Can you work these out from the model? Positions are in its coordinate system, mm. Face numbers are marked on the shaded views. A direction names the side the tool comes from. Give positions to 0.01 mm unless a question says otherwise; leave off trailing zeros. Order: outer loops, then holes, each group sorted by start corner. A loop starts at its lowest first (then second) coordinate and runs counter-clockwise, first axis right, second up. Notation, with made-up numbers: (82, -32) -> (106, -32) arc R19 cw to (106, 3) -> close; hole circle Ø8 at (-20, 23). An arc over 180 degrees is marked (long way). Answer as a JSON object with one key per item and string values.
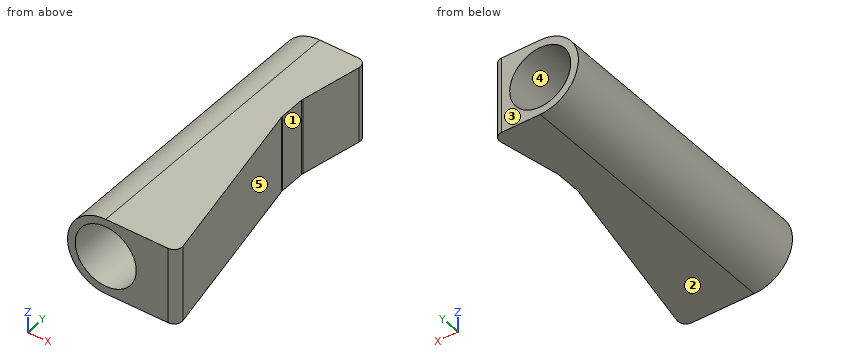
```python
from build123d import *

# Parameters (mm, degrees)
SKETCH1_R           = 14.2875
SKETCH1_R_2         = 11.4125
BOSS_EXTRUDE1_DEPTH = 152.4
SKETCH2_W           = 28.575
SKETCH2_H           = 152.4
BOSS_EXTRUDE2_DEPTH = 12.7
BOSS_EXTRUDE3_DEPTH = 152.4
CUT_EXTRUDE1_DEPTH  = 29.575
FILLET1_R           = 3
SKETCH6_W           = 50
SKETCH6_H           = 45
CUT_EXTRUDE2_DEPTH  = 82
FILLET2_R           = 3


with BuildPart() as part:
    # Sketch1 → Boss-Extrude1 (new body)
    with BuildSketch(Plane(origin=(0, 0, 0), x_dir=(1, 0, 0), z_dir=(0, 1, 0))):
        Circle(SKETCH1_R)
        Circle(SKETCH1_R_2, mode=Mode.SUBTRACT)
    extrude(amount=BOSS_EXTRUDE1_DEPTH)



with BuildPart() as body_2:
    # Sketch2 → Boss-Extrude2 (new body)
    with BuildSketch(Plane(origin=(14.2875, 0, 0), x_dir=(0, 0, -1), z_dir=(1, 0, 0))):
        with Locations((0, 76.2)):
            Rectangle(SKETCH2_W, SKETCH2_H)
    extrude(amount=BOSS_EXTRUDE2_DEPTH)


with BuildPart() as part_1:
    add(part.part)

    add(body_2.part)  # Boss-Extrude3 merges body 2
    # Sketch3 → Boss-Extrude3 (add, through all)
    with BuildSketch(Plane(origin=(0, 152.4, 0), x_dir=(1, 0, 0), z_dir=(0, 1, 0))):
        with BuildLine():
            Line((14.2875, -14.2875), (0, -14.2875))
            ThreePointArc((0, -14.2875), (14.2875, 0), (0, 14.2875))
            Line((0, 14.2875), (14.2875, 14.2875))
            Line((14.2875, 14.2875), (26.9875, 14.2875))
            Line((26.9875, 14.2875), (26.9875, -14.2875))
            Line((26.9875, -14.2875), (14.2875, -14.2875))
        make_face()
    extrude(amount=-BOSS_EXTRUDE3_DEPTH)

    # Sketch5 → Cut-Extrude1 (cut, through all)
    with BuildSketch(Plane.XY.offset(14.2875)):
        Polygon((26.9875, 0), (12.897222949, 71.2), (12.897222949, 81.2), (26.9875, 152.4), align=None)
    extrude(amount=-CUT_EXTRUDE1_DEPTH, mode=Mode.SUBTRACT)

    # Fillet1
    fillet1_edges = [part_1.edges().sort_by_distance(p)[0] for p in [
        (26.9875, 0, 0),
        (26.9875, 152.4, 0),
        (12.897222949, 71.2, 0),
        (12.897222949, 81.2, 0),
    ]]
    fillet(fillet1_edges, radius=FILLET1_R)

    # Sketch6 → Cut-Extrude2 (cut)
    with BuildSketch(Plane.XY.offset(14.2875)):
        with Locations((9.7125, 129.9)):
            Rectangle(SKETCH6_W, SKETCH6_H)
    extrude(amount=-CUT_EXTRUDE2_DEPTH, mode=Mode.SUBTRACT)

    # Fillet2
    fillet2_edges = [part_1.edges().sort_by_distance(p)[0] for p in [
        (18.082128268, 107.4, 0),
    ]]
    fillet(fillet2_edges, radius=FILLET2_R)


solid = part_1.part
```
1. If we section it at A-A on z = 0: Please give me the cut outline in (x, y).
Worked answers:
{"outline": "(-14.29, 0) -> (-11.41, 0) -> (-11.41, 107.4) -> (-14.29, 107.4) -> close; (11.41, 0) -> (23.34, 0) arc R3 ccw to (26.28, 3.58) -> (12.95, 70.91) arc R3 cw to (12.9, 71.49) -> (12.9, 80.91) arc R3 cw to (12.95, 81.49) -> (17.37, 103.82) arc R3 ccw to (14.43, 107.4) -> (11.41, 107.4) -> close"}
2. If we mould it in two halves opening along Y, with no side actions, what happens to the marked faces 3, 4 and 5? For each: +Y half, -Y half, draft (parallel to the pull), parting line (faces both ways), or undercut.
Worked answers:
{"face 3": "+Y half", "face 4": "draft", "face 5": "undercut"}
3. If we section it at C-C on y = 91.5: Please give me the cut outline in (x, z) (1 decimal), then the cut area to 3 significant figures.
Worked answers:
{"outline": "(0, -14.3) -> (14.9, -14.3) -> (14.9, 14.3) -> (0, 14.3) arc R14.3 ccw to start; hole circle Ø22.8 at (0, 0)", "area": "338 mm²"}
4. If we section it at D-D on x = -2.5: Please give me the cut outline in (y, z), then the cut area to 3 significant figures.
Worked answers:
{"outline": "(0, -14.07) -> (107.4, -14.07) -> (107.4, -11.14) -> (0, -11.14) -> close; (0, 11.14) -> (107.4, 11.14) -> (107.4, 14.07) -> (0, 14.07) -> close", "area": "630 mm²"}
5. Will these pins go through, and if not, where does the flat tip stop? pin 1 Ø5 at (x, z) = (-7.5, 1.5) entering from +Y; pin 2 Ø4 at (y, z) = (27, 11.5) entering from -X; pin 3 Ø5 at (y, z) = (60, 9.5) entering from -X; pin 4 Ø8 at (y, z) = (62.5, 2) entering from -X.
Worked answers:
{"pin 1": "through", "pin 2": "x = -10.67", "pin 3": "x = -12.46", "pin 4": "x = -14.29"}
6. If we section it at B-B on x = -8: Please give me the cut outline in (y, z), then the cut area to 3 significant figures.
Worked answers:
{"outline": "(0, -11.84) -> (107.4, -11.84) -> (107.4, -8.14) -> (0, -8.14) -> close; (0, 8.14) -> (107.4, 8.14) -> (107.4, 11.84) -> (0, 11.84) -> close", "area": "794 mm²"}
7. For the marked faces 1 and 2, which set-ups out of +Z, -Z, +X, -X, +Y, -Y let a thin tool reach every point of the face, with its end or its side?
Worked answers:
{"face 1": "+Z, -Z, +X", "face 2": "-Z, +X, -X, +Y, -Y"}
8. Please list where these lines run through material, in increasing order: L1, parallel to X at y = 13, z = 4.25; L2, parallel to Z at x = 8, y = 45.5; L3, parallel to X at y = 75, z = 0.
Worked answers:
{"L1": "-13.64 to -10.59, 10.59 to 24.41", "L2": "-14.29 to -8.14, 8.14 to 14.29", "L3": "-14.29 to -11.41, 11.41 to 12.9"}
